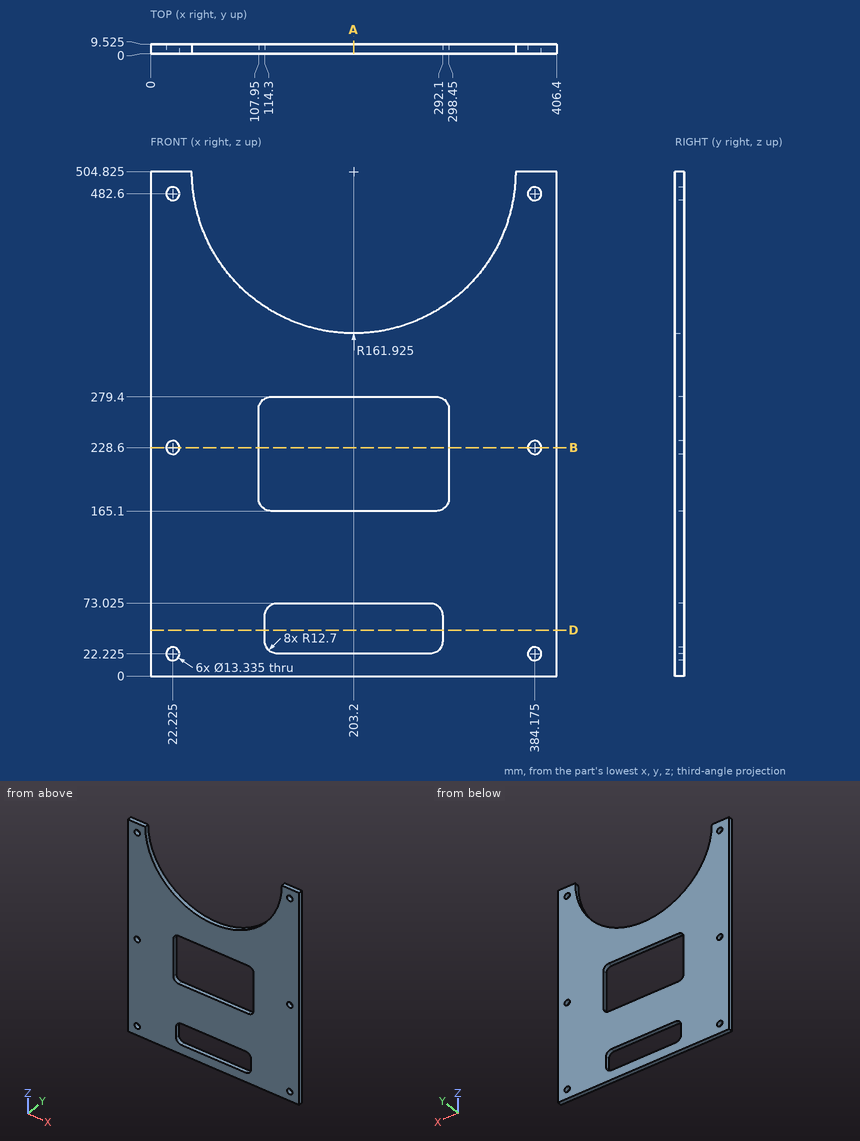
Study the drawing (mm; zero at the part's minimum x, y, z) and answer. Give positions to 0.01 mm unless a question says otherwise; leave off trailing zeros. Write each loop counter-clockwise with the first axis right and the second up, starting at its lowest first coordinate (ties: lowest second). Pieces come first, ordered by that corner, then holes. Notation, with made-up numbers: (28.5, 76) -> (63.5, 76) arc R25 ccw to (63.5, 107) -> close; hole circle Ø10 at (89, 1). An arc over 180 degrees is marked (long way). Answer as a JSON object with one key per item and string values. Group by question number.
1) Consider L1, parallel to X at y = 3.5, z = 228.6; L2, parallel to X at y = 6.5, z = 178; L3, parallel to Z at x = 125.5, y = 6.75. Determine where each line is inside the solid, lowest interval first. Write a range as from..to.
2) Each of these flat-tipped pins is pushed along its axis until it touches: P1, Ø4, axis at x = 178, y = 1, coming from the +Z side; P2, Ø10.5, axis at x = 384.175, z = 22.225, coming from the +Y side; P3, Ø5, axis at x = 104, y = 7, coming from the +Z side; P4, Ø3, axis at x = 93, y = 7, coming from the +Z side. Where does it stop, or does it pass through?
3) Find section B-B (z = 228.6). Count the separate pieces of the cut face and the enclosed holes in it, and give its area (3 significant figures).
4) Find section D-D (z = 46). Write down the section's boundary in (x, y) (3 decimals), and give its area (3 significant figures).
5) Find section A-A (x = 203.2). Write down the section's boundary in (y, z) (3 decimals).
Values follow:
{
 "1": {"L1": "x = 0..15.56, 28.89..107.95, 298.45..377.51, 390.84..406.4", "L2": "x = 0..107.95, 298.45..406.4", "L3": "z = 0..22.31, 72.94..165.1, 279.4..362.76"},
 "2": {"P1": "stops at z = 345.2", "P2": "passes through", "P3": "stops at z = 378.82", "P4": "stops at z = 387.6"},
 "3": {"separate pieces": "4", "enclosed holes": "0", "area": "1,800 mm2"},
 "4": {"outline": "(0, 0) -> (114.3, 0) -> (114.3, 9.525) -> (0, 9.525) -> close; (292.1, 0) -> (406.4, 0) -> (406.4, 9.525) -> (292.1, 9.525) -> close", "area": "2,180 mm2"},
 "5": {"outline": "(0, 0) -> (9.525, 0) -> (9.525, 22.225) -> (0, 22.225) -> close; (0, 73.025) -> (9.525, 73.025) -> (9.525, 165.1) -> (0, 165.1) -> close; (0, 279.4) -> (9.525, 279.4) -> (9.525, 342.9) -> (0, 342.9) -> close"}
}
